Could you check a few things on this model? Use its own coordinates, in mm. A direction names the side the tool comes from. Give positions to 0.01 mm unless a question says otherwise; leave off trailing zeros. Loops run counter-clockwise (first coordinate to the right, second up) from the corner with the lowest first, then second, coordinate; pieces in that order, holes last. Notation, with made-up numbers: (-32.75, -1) - (-26.75, -1) arc R7 cw to (-26.75, 12) - close; hole circle Ø10 at (-20.5, -31.75). An arc over 180 degrees is marked (long way). Use CSV: the item, a comma, the result in double quotes.
from build123d import *

# Parameters (mm, degrees)
BOSS_EXTRUDE1_DEPTH           = 11.1125
CHAMFER1_SIZE                 = 10.16
TAP_DRILL_FOR_8_32_TAP1_D     = 3.4544
TAP_DRILL_FOR_8_32_TAP1_DEPTH = 12.7
TAP_DRILL_FOR_8_32_TAP1_TIP   = 1.037806461
SKETCH27_R                    = 4.7625
CUT_EXTRUDE1_DEPTH            = 12.1125


with BuildPart() as part:
    # Sketch1 → Boss-Extrude1 (new body)
    with BuildSketch(Plane(origin=(0, 0, 0), x_dir=(1, 0, 0), z_dir=(0, 1, 0))):
        with BuildLine():
            Line((-26.083081673, -38.1), (-13.335, 0))
            ThreePointArc((-13.335, 0), (0, 13.335), (13.335, 0))
            Line((13.335, 0), (26.083081673, -38.1))
            Line((26.083081673, -38.1), (38.1, -38.1))
            Line((38.1, -38.1), (38.1, 38.1))
            Line((38.1, 38.1), (-38.1, 38.1))
            Line((-38.1, 38.1), (-38.1, -38.1))
            Line((-38.1, -38.1), (-26.083081673, -38.1))
        make_face()
    extrude(amount=BOSS_EXTRUDE1_DEPTH)

    # Chamfer1
    chamfer1_edges = [part.edges().sort_by_distance(p)[0] for p in [
        (19.709040837, 11.1125, 19.05),
        (-19.709040837, 11.1125, 19.05),
        (0, 11.1125, -13.335),
    ]]
    chamfer(chamfer1_edges, length=CHAMFER1_SIZE)

    # Tap Drill for #8-32 Tap1
    with Locations(Plane(origin=(0, 5.55625, -38.1), x_dir=(-1, 0, 0), z_dir=(0, 0, -1))):
        with Locations((0, 0)):
            Hole(TAP_DRILL_FOR_8_32_TAP1_D / 2, depth=TAP_DRILL_FOR_8_32_TAP1_DEPTH)
            with Locations((0, 0, -(TAP_DRILL_FOR_8_32_TAP1_DEPTH + TAP_DRILL_FOR_8_32_TAP1_TIP / 2))):  # 118° drill point
                Cone(0, TAP_DRILL_FOR_8_32_TAP1_D / 2, TAP_DRILL_FOR_8_32_TAP1_TIP, mode=Mode.SUBTRACT)

    # Sketch27 → Cut-Extrude1 (cut, through all)
    with BuildSketch(Plane(origin=(0, 11.1125, 0), x_dir=(1, 0, 0), z_dir=(0, 1, 0))):
        with Locations((0, 30.7975)):
            Circle(SKETCH27_R)
    extrude(amount=-CUT_EXTRUDE1_DEPTH, mode=Mode.SUBTRACT)


solid = part.part
1) We'd pull the mould along Y, two halves only. Please class faces 4 (the conical face through (-0.33, 2.72, -15.1)), 5 (the flat face through (-1, 0, -17)), 6 (the cylindrical face through (-0.29, 0.47, -13.33)), 7 (the conical face through (0.04, 5.85, -24.54)): +Y half, -Y half, draft (parallel to the pull), parting line (faces both ways), or undercut.
Answer below:
face 4,"+Y half"
face 5,"-Y half"
face 6,"draft"
face 7,"undercut"
2) Suppose I cut it at A-A (z = 18). Please give me the cut outline in (x, y).
Answer below:
outline,"(-38.1, 0) - (-19.36, 0) - (-19.36, 0.95) - (-30.07, 11.11) - (-38.1, 11.11) - close; (19.36, 0) - (38.1, 0) - (38.1, 11.11) - (30.07, 11.11) - (19.36, 0.95) - close"
3) Suppose I cut it at C-C (x = 32.5). Please give me the cut outline in (y, z), plus the area to 3 significant figures.
Answer below:
outline,"(0, -38.1) - (11.11, -38.1) - (11.11, 25.26) - (7.04, 38.1) - (0, 38.1) - close"
area,"821 mm2"
4) Suppose I cut it at D-D (x = -29). Please give me the cut outline in (y, z).
Answer below:
outline,"(0, -38.1) - (11.11, -38.1) - (11.11, 14.8) - (3.72, 38.1) - (0, 38.1) - close"
5) I need wall thicknesses on line 1 along Y through (x, z) = (0, -36); line 2 along Z through (x, y) = (-3.5, 7.75); line 3 along X through (y, z) = (5, 23.5). Which ranges of each line are inside material? Lowest first, please.
Answer below:
line 1,"y = 0 to 3.83, 7.28 to 11.11"
line 2,"z = -38.1 to -34.03, -27.57 to -19.83"
line 3,"x = -38.1 to -25.47, 25.47 to 38.1"
6) Which directions (+Z, -Z, +X, -X, +Y, -Y) give clear straight access to the entire face, cutting with the end or side of a thin tool? Please do faces 1 (the flat face through (-25.23, 6.1, 19.32)), 2 (the flat face through (19.62, 0.47, 18.78)), 3 (the cylindrical face through (1.647, 6.075, -25.766)).
Answer below:
face 1,"+Z, +Y"
face 2,"+Z, +Y, -Y"
face 3,"-Z"
7) I'm going to push flat-ended pins straight in: P1, Ø4.5, axis at x = 0, y = 5.56, coming from the +Z side; P2, Ø10, axis at x = -14, z = 9.5, coming from the -Y side; P3, Ø3, axis at x = -5, y = 10, coming from the +Z side. Where does each tip first touch, or does it pass through?
Answer below:
P1,"stops at z = -15.69"
P2,"stops at y = 0"
P3,"stops at z = -20.23"
